The model under review builds one solid part; all positions refer to its coordinate system, in mm. A direction names the side the tool comes from. Coordinates: 2 decimals unless noted, no trailing zeros. Write each loop counter-clockwise with the first axis right and the second up, starting at its lowest first coordinate (ties: lowest second). Pieces come first, ordered by that corner, then holes. Notation, with made-up numbers: (-22, -27.5) - (34, -27.5) arc R20 ccw to (34, -8.5) - close; hole circle Ø9 at (70, 73.25). An arc over 180 degrees is marked (long way). Return JSON: item names as keys, results as strings. Group by question number.
(1) We need section C-C on x = 6. State the section outline as (y, z) points (3 decimals), then the cut area to 3 significant figures.
(2) Draft analysis for pull direction Y (two halves, no side actions). For faces 3 (the face through (15.155, 3.283, 0.488)), 4 (the face through (-0.27, -8.17, -0.38)), 5 (the face through (0, -9, -19.05)), state which applies: released by +Y, released by -Y, zero draft, split by the parting line, or undercut.
(3) To check wall thickness, follow L1, parallel to X at y = -9.2, z = -12.7; L2, parallel to Z at x = 10, y = -5.25; L3, parallel to Y at x = 8, z = -3.75 (3 decimals). State the ranges of each line that lie inside material, in increasing order. Write a range as from..to.
(4) For pin 1 Ø5 at (x, y) = (-3, -2) entering from -Z; pin 2 Ø4 at (x, y) = (-12.7, 3.175) entering from -Z, all flat-tipped, find the tip position at first contact; note any pin that passes through.
(5) We need section B-B on x = -12.7. State the section outline as (y, z) points (3 decimals), then the cut area to 3 significant figures.
(6) We need section A-A on z = -12.7. State the section outline as (x, y) points (3 decimals), then the cut area to 3 significant figures.
(7) Tool access review of faces 1 (the face through (0, 1, 0)), 2 (the face through (-19.202, -9, -4)): name each direction out of +Z, -Z, +X, -X, +Y, -Y from which nothing blocks a thin tool from reaching the whole face with its end or side.
(8) We need section D-D on y = -6.25. State the section outline as (x, z) points.
```python
from build123d import *

# Parameters (mm, degrees)
SKETCH1_W                    = 38.4048
SKETCH1_H                    = 19.05
BOSS_EXTRUDE1_DEPTH          = 0.9906
F_10_0_1935_DIAMETER_HOLE1_D = 4.9149
SKETCH5_W                    = 38.4048
SKETCH5_H                    = 0.9906
BOSS_EXTRUDE2_DEPTH          = 19.05
F_10_0_1935_DIAMETER_HOLE2_D = 4.9149
FILLET1_R                    = 1.27


with BuildPart() as part:
    # Sketch1 → Boss-Extrude1 (new body)
    with BuildSketch(Plane.XY):
        Rectangle(SKETCH1_W, SKETCH1_H)
    extrude(amount=BOSS_EXTRUDE1_DEPTH)

    # #10 (0.1935) Diameter Hole1 (through all)
    with Locations(Plane.XY.offset(0.9906)):
        with Locations((-12.7, 3.175), (12.7, 3.175)):
            Hole(F_10_0_1935_DIAMETER_HOLE1_D / 2)

    # Sketch5 → Boss-Extrude2 (add)
    with BuildSketch(Plane(origin=(0, 0, 0), x_dir=(-1, 0, 0), z_dir=(0, 0, -1))):
        with Locations((0, -9.0297)):
            Rectangle(SKETCH5_W, SKETCH5_H)
    extrude(amount=BOSS_EXTRUDE2_DEPTH)

    # #10 (0.1935) Diameter Hole2 (through all)
    with Locations(Plane(origin=(0, -8.5344, 0), x_dir=(1, 0, 0), z_dir=(0, 1, 0))):
        with Locations((-12.7, 12.7), (12.7, 12.7)):
            Hole(F_10_0_1935_DIAMETER_HOLE2_D / 2)

    # Fillet1
    fillet1_edges = [part.edges().sort_by_distance(p)[0] for p in [
        (0, -8.5344, 0),
        (0, -9.525, 0.9906),
    ]]
    fillet(fillet1_edges, radius=FILLET1_R)


solid = part.part
```
Ans:
{
 "1": {"outline": "(-9.525, -19.05) - (-8.534, -19.05) - (-8.534, -1.27) arc R1.27 cw to (-7.264, 0) - (9.525, 0) - (9.525, 0.991) - (-8.255, 0.991) arc R1.27 ccw to (-9.525, -0.279) - close", "area": "37.7 mm²"},
 "2": {"face 3": "undercut", "face 4": "released by +Y", "face 5": "zero draft"},
 "3": {"L1": "-19.2..-15.16, -10.24..10.24, 15.16..19.2", "L2": "0..0.99", "L3": "-9.525..-8.534"},
 "4": {"pin 1": "z = 0", "pin 2": "through"},
 "5": {"outline": "(-9.525, -19.05) - (-8.534, -19.05) - (-8.534, -15.157) - (-9.525, -15.157) - close; (-9.525, -10.243) - (-8.534, -10.243) - (-8.534, -1.27) arc R1.27 cw to (-7.264, 0) - (0.718, 0) - (0.718, 0.991) - (-8.255, 0.991) arc R1.27 ccw to (-9.525, -0.279) - close; (5.632, 0) - (9.525, 0) - (9.525, 0.991) - (5.632, 0.991) - close", "area": "28.0 mm²"},
 "6": {"outline": "(-19.202, -9.525) - (-15.157, -9.525) - (-15.157, -8.534) - (-19.202, -8.534) - close; (-10.243, -9.525) - (10.243, -9.525) - (10.243, -8.534) - (-10.243, -8.534) - close; (15.157, -9.525) - (19.202, -9.525) - (19.202, -8.534) - (15.157, -8.534) - close", "area": "28.3 mm²"},
 "7": {"face 1": "-Z, +X, -X, +Y", "face 2": "+Z, -Z, -X, +Y, -Y"},
 "8": {"outline": "(-19.2, 0) - (19.2, 0) - (19.2, 0.99) - (-19.2, 0.99) - close"}
}
